The listing builds one solid part. Answer for the finished solid, in the listing's coordinates (mm). Coordinates: 2 decimals unless noted, no trailing zeros. Write each loop counter-clockwise with the first axis right and the second up, starting at its lowest first coordinate (ties: lowest second). Pieces come first, ordered by that corner, then holes.
from build123d import *

# Parameters (mm, degrees)
ESQUISSE1_W                          = 192
ESQUISSE1_H                          = 292
BOSS_EXTRU_1_DEPTH                   = 4
ENL_V_MAT_EXTRU_17_DEPTH             = 330.683341579
R_P_TITION_LIN_AIRE2_COUNT           = 2
R_P_TITION_LIN_AIRE2_PITCH           = 141.43
ESQUISSE5_R                          = 4
BOSS_EXTRU_2_DEPTH                   = 3
ESQUISSE6_R                          = 1.5
ENL_V_MAT_EXTRU_18_DEPTH             = 6
ESQUISSE7_R                          = 1.5
ENL_V_MAT_EXTRU_19_DEPTH             = 6
R_P_TITION_LIN_AIRE5_COUNT           = 2
R_P_TITION_LIN_AIRE5_PITCH           = 130.815
ESQUISSE10_R                         = 1.5
ENL_V_MAT_EXTRU_20_DEPTH             = 6
ESQUISSE9_R                          = 4
BOSS_EXTRU_3_DEPTH                   = 3
ESQUISSE11_R                         = 1.5
ENL_V_MAT_EXTRU_21_DEPTH             = 6
R_P_TITION_LIN_AIRE6_COUNT           = 2
R_P_TITION_LIN_AIRE6_PITCH           = 31.82
R_P_TITION_LIN_AIRE7_COUNT           = 2
R_P_TITION_LIN_AIRE7_PITCH           = 130.815
R_P_TITION_LIN_AIRE7_COPY_1_SKETCH_R = 4
R_P_TITION_LIN_AIRE7_COPY_1_DEPTH    = 3
R_P_TITION_LIN_AIRE7_COPY_2_SKETCH_R = 1.5
R_P_TITION_LIN_AIRE7_COPY_2_DEPTH    = 6
ESQUISSE14_R                         = 2.5
ENL_V_MAT_EXTRU_22_DEPTH             = 330.683341579
CONG_2_R                             = 5


with BuildPart() as part:
    # Esquisse1 → Boss.-Extru.1 (new body)
    with BuildSketch(Plane.XY):
        with Locations((77.321557543, 134.418871343)):
            Rectangle(ESQUISSE1_W, ESQUISSE1_H)
    extrude(amount=BOSS_EXTRU_1_DEPTH)

    # Esquisse4 → Enlèv. mat.-Extru.17 (cut, through all)
    with BuildSketch(Plane.XY.offset(4)):
        Polygon((77.321557543, 276.118871343), (6.610879425, 205.408193225), (77.321557543, 134.697515106), (148.032235662, 205.408193225), align=None)
    enl_v_mat_extru_17 = extrude(amount=-ENL_V_MAT_EXTRU_17_DEPTH, mode=Mode.SUBTRACT)

    # Répétition linéaire2: Enlèv. mat.-Extru.17 ×2
    with Locations(*[(0, -i * R_P_TITION_LIN_AIRE2_PITCH, 0) for i in range(1, R_P_TITION_LIN_AIRE2_COUNT)]):
        add(enl_v_mat_extru_17, mode=Mode.SUBTRACT)

    # Esquisse5 → Boss.-Extru.2 (add)
    with BuildSketch(Plane.XY.offset(4)):
        with Locations(Location((61.411654967, 270.815570484, 0), (0, 0, 180))):
            Circle(ESQUISSE5_R)
        with Locations(Location((93.23146012, 270.815570484, 0), (0, 0, 180))):
            Circle(ESQUISSE5_R)
    boss_extru_2 = extrude(amount=BOSS_EXTRU_2_DEPTH)

    # Esquisse6 → Enlèv. mat.-Extru.18 (cut)
    with BuildSketch(Plane.XY.offset(7)):
        with Locations((61.411654967, 270.815570484)):
            Circle(ESQUISSE6_R)
    enl_v_mat_extru_18 = extrude(amount=-ENL_V_MAT_EXTRU_18_DEPTH, mode=Mode.SUBTRACT)

    # Esquisse7 → Enlèv. mat.-Extru.19 (cut)
    with BuildSketch(Plane.XY.offset(7)):
        with Locations((93.23146012, 270.815570484)):
            Circle(ESQUISSE7_R)
    extrude(amount=-ENL_V_MAT_EXTRU_19_DEPTH, mode=Mode.SUBTRACT)

    # Répétition linéaire5: Boss.-Extru.2, Enlèv. mat.-Extru.18 ×2
    with Locations(*[(0, -i * R_P_TITION_LIN_AIRE5_PITCH, 0) for i in range(1, R_P_TITION_LIN_AIRE5_COUNT)]):
        add(boss_extru_2)
        add(enl_v_mat_extru_18, mode=Mode.SUBTRACT)

    # Esquisse10 → Enlèv. mat.-Extru.20 (cut)
    with BuildSketch(Plane.XY.offset(7)):
        with Locations((93.23146012, 140.000570484)):
            Circle(ESQUISSE10_R)
    extrude(amount=-ENL_V_MAT_EXTRU_20_DEPTH, mode=Mode.SUBTRACT)

    # Esquisse9 → Boss.-Extru.3 (add)
    with BuildSketch(Plane.XY.offset(4)):
        with Locations(Location((93.23146012, 129.385570484, 0), (0, 0, 180))):
            Circle(ESQUISSE9_R)
    boss_extru_3 = extrude(amount=BOSS_EXTRU_3_DEPTH)

    # Esquisse11 → Enlèv. mat.-Extru.21 (cut)
    with BuildSketch(Plane.XY.offset(7)):
        with Locations((93.23146012, 129.385570484)):
            Circle(ESQUISSE11_R)
    enl_v_mat_extru_21 = extrude(amount=-ENL_V_MAT_EXTRU_21_DEPTH, mode=Mode.SUBTRACT)

    # Répétition linéaire6: Boss.-Extru.3, Enlèv. mat.-Extru.21 ×2
    with Locations(*[(-i * R_P_TITION_LIN_AIRE6_PITCH, 0, 0) for i in range(1, R_P_TITION_LIN_AIRE6_COUNT)]):
        add(boss_extru_3)
        add(enl_v_mat_extru_21, mode=Mode.SUBTRACT)

    # Répétition linéaire7: Boss.-Extru.3, Enlèv. mat.-Extru.21 ×2
    with Locations(*[(0, -i * R_P_TITION_LIN_AIRE7_PITCH, 0) for i in range(1, R_P_TITION_LIN_AIRE7_COUNT)]):
        add(boss_extru_3)
        add(enl_v_mat_extru_21, mode=Mode.SUBTRACT)

    # Répétition linéaire7 copy 1 sketch → Répétition linéaire7 copy 1 (add)
    with BuildSketch(Plane(origin=(-31.82, -130.815, 4), x_dir=(1, 0, 0), z_dir=(0, 0, 1))):
        with Locations(Location((93.23146012, 129.385570484, 0), (0, 0, 180))):
            Circle(R_P_TITION_LIN_AIRE7_COPY_1_SKETCH_R)
    extrude(amount=R_P_TITION_LIN_AIRE7_COPY_1_DEPTH)

    # Répétition linéaire7 copy 2 sketch → Répétition linéaire7 copy 2 (cut)
    with BuildSketch(Plane(origin=(-31.82, -130.815, 7), x_dir=(1, 0, 0), z_dir=(0, 0, 1))):
        with Locations((93.23146012, 129.385570484)):
            Circle(R_P_TITION_LIN_AIRE7_COPY_2_SKETCH_R)
    extrude(amount=-R_P_TITION_LIN_AIRE7_COPY_2_DEPTH, mode=Mode.SUBTRACT)

    # Esquisse14 → Enlèv. mat.-Extru.22 (cut, through all)
    with BuildSketch(Plane.XY.offset(4)):
        with Locations((1.321557543, 8.418871343)):
            Circle(ESQUISSE14_R)
        with Locations((153.321557543, 8.418871343)):
            Circle(ESQUISSE14_R)
        with Locations((153.321557543, 260.418871343)):
            Circle(ESQUISSE14_R)
        with Locations((1.321557543, 260.418871343)):
            Circle(ESQUISSE14_R)
    extrude(amount=-ENL_V_MAT_EXTRU_22_DEPTH, mode=Mode.SUBTRACT)

    # Congé2
    cong_2_edges = [part.edges().sort_by_distance(p)[0] for p in [
        (6.610879425, 205.408193225, 2),
        (77.321557543, 276.118871343, 2),
        (148.032235662, 205.408193225, 2),
        (77.321557543, 134.697515106, 2),
        (6.610879425, 63.978193225, 2),
        (77.321557543, 134.688871343, 2),
        (148.032235662, 63.978193225, 2),
        (77.321557543, -6.732484894, 2),
    ]]
    fillet(cong_2_edges, radius=CONG_2_R)


solid = part.part
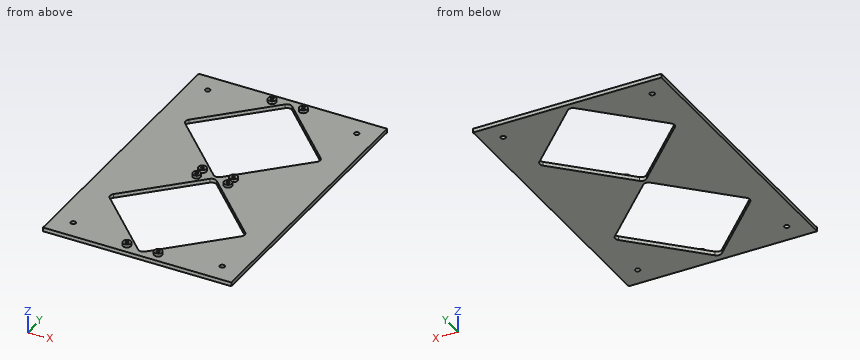
1. Section D-D on y = 157 is taken. Give the vertices of the cut face in (x, z), then the cut area to 3 significant figures.
Results found:
outline: (-18.68, 0) - (55.02, 0) - (55.02, 4) - (-18.68, 4) - close; (99.62, 0) - (173.32, 0) - (173.32, 4) - (99.62, 4) - close
area: 590 mm2
2. Section C-C on x = 51 is taken. Give the vertices of the cut face in (y, z), then the cut area to 3 significant figures.
Results found:
outline: (-11.58, 0) - (19.59, 0) - (19.59, 4) - (-11.58, 4) - close; (108.37, 0) - (161.02, 0) - (161.02, 4) - (108.37, 4) - close; (249.8, 0) - (280.42, 0) - (280.42, 4) - (249.8, 4) - close
area: 458 mm2
3. Section A-A on y = 219 is taken. Give the vertices of the cut face in (x, z), then the cut area to 3 significant figures.
Results found:
outline: (-18.68, 0) - (20.2, 0) - (20.2, 4) - (-18.68, 4) - close; (134.44, 0) - (173.32, 0) - (173.32, 4) - (134.44, 4) - close
area: 311 mm2
4. Section B-B on z = 5.25 is taken. State how many separate pieces and enclosed holes the cut face has, then the cut area to 3 significant figures.
Results found:
separate pieces: 8
enclosed holes: 8
area: 346 mm2
5. Find the intervals of material crossed by L1, parallel to Y at x = 98, z = 1.25; L2, parallel to Y at x = 41, z = 2; L3, parallel to X at y = 262.5, z = 1.25, in increasing order.
Results found:
L1: y = -11.58 to 13.95, 114.01 to 155.38, 255.44 to 280.42
L2: y = -11.58 to 29.59, 98.37 to 171.02, 239.8 to 280.42
L3: x = -18.68 to -0.06, 2.71 to 63.7, 90.94 to 151.94, 154.71 to 173.32
6. Flat-ended cylindrical pins translate along their axes: P1, Ø1.5, axis at y = 160, z = 5, coming from the -X side; P2, Ø1.8, axis at x = 93.23, y = -1.43, coming from the +Z side; P3, Ø2.5, axis at x = 93, y = -1, coming from the +Z side; P4, Ø5, axis at x = 3.5, y = 213, coming from the +Z side. Find the tip coordinate at first contact, or state that the pin passes through.
Results found:
P1: passes through
P2: stops at z = 1
P3: stops at z = 7
P4: stops at z = 4
